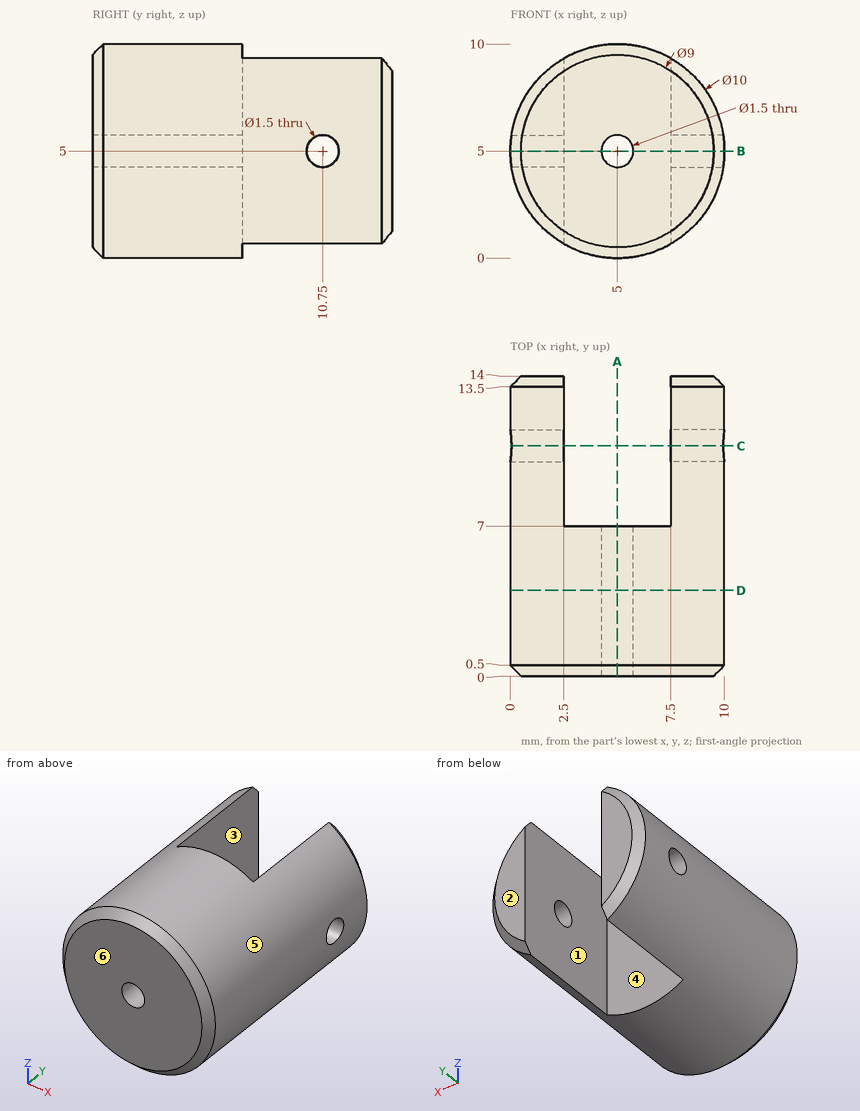
For this review, use the dimensioned drawing (mm, ordinates from the lowest corner) and the shaded views. A direction names the side the tool comes from. Coordinates: 2 decimals unless noted, no trailing zeros. Loops run counter-clockwise (first coordinate to the right, second up) from the corner with the lowest first, then second, coordinate; pieces in that order, holes last.
1. For line 1 (Z direction, x = 0.6, y = 10.75); line 2 (X direction, y = 8.25, z = 2.5); line 3 (X direction, y = 9.5, z = 8), list the stretches that pass through material, from the lowest coordinate up.
2. Insertion check: P1, Ø3, axis at x = 5.5, z = 1.5, coming from the +Y side; P2, Ø2, axis at x = 7, y = 9, coming from the +Z side; P3, Ø1.5, axis at x = 3, y = 8.5, coming from the -Z side; P4, Ø0.9, axis at y = 10.75, z = 5, coming from the +X side. Each pin has a flat end and moves straight along its axis. Give the tip position at first contact, or say it passes through.
3. Add section C-C, the plane y = 10.75. Give the boundary of the cut face in (x, z).
4. Add section D-D, the plane y = 4. Give the boundary of the cut face in (x, z).
5. Mouldability with a two-part tool opening along X and no side actions: class the marked faces 3, 4, 5 and 6 as +X half, -X half, draft (parallel to the pull), parting line (faces both ways), or undercut.
6. Add section A-A, the plane x = 5. Give the boundary of the cut face in (y, z), then the cut area to 4 significant figures.
7. Add section B-B, the plane z = 5. Give the boundary of the cut face in (x, y), then the cut area to 3 significant figures.
8. For the marked faces 1 and 2, list the 3-axis set-ups (+Z, -Z, +X, -X, +Y, -Y) from which the entire face can be reached by the end or side of a thin tool; tool diameter is ignored.
Result:
1. line 1: z = 2.63 to 4.25, 5.75 to 7.37
1. line 2: x = 0.67 to 2.5, 7.5 to 9.33
1. line 3: x = 1 to 2.5, 7.5 to 9
2. P1: stops at y = 7
2. P2: stops at z = 9.33
2. P3: stops at z = 0.67
2. P4: passes through
3. outline: (0.06, 4.25) arc R5 ccw to (2.5, 0.67) - (2.5, 4.25) - close; (0.06, 5.75) - (2.5, 5.75) - (2.5, 9.33) arc R5 ccw to start; (7.5, 0.67) arc R5 ccw to (9.94, 4.25) - (7.5, 4.25) - close; (7.5, 5.75) - (9.94, 5.75) arc R5 ccw to (7.5, 9.33) - close
4. outline: circle Ø10 at (5, 5); hole circle Ø1.5 at (5, 5)
5. face 3: undercut
5. face 4: undercut
5. face 5: parting line
5. face 6: draft
6. outline: (0, 0.5) - (0.5, 0) - (7, 0) - (7, 4.25) - (0, 4.25) - close; (0, 5.75) - (7, 5.75) - (7, 10) - (0.5, 10) - (0, 9.5) - close
6. area: 59.25 mm2
7. outline: (0, 0.5) - (0.5, 0) - (4.25, 0) - (4.25, 7) - (2.5, 7) - (2.5, 10) - (0, 10) - close; (0, 11.5) - (2.5, 11.5) - (2.5, 14) - (0.5, 14) - (0, 13.5) - close; (5.75, 0) - (9.5, 0) - (10, 0.5) - (10, 10) - (7.5, 10) - (7.5, 7) - (5.75, 7) - close; (7.5, 11.5) - (10, 11.5) - (10, 13.5) - (9.5, 14) - (7.5, 14) - close
7. area: 86.5 mm2
8. face 1: +Z, -Z, +Y
8. face 2: +Z, -Z, +X, -X, +Y
